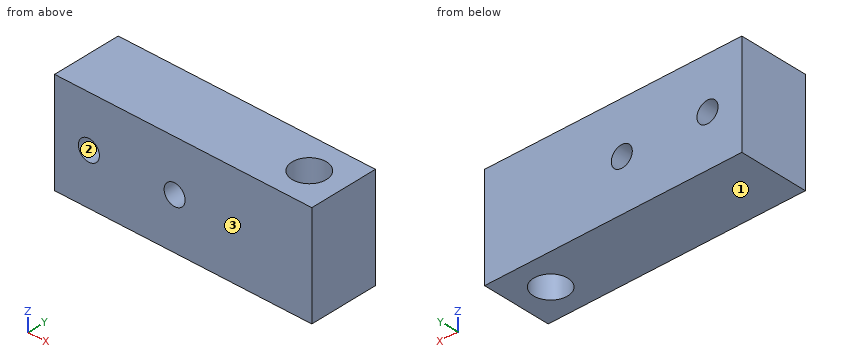
Autodesk Inventor part; units mm, degrees
ref_plane "YZ Plane" through (0, 0, 0) normal (1, 0, 0) x (0, 1, 0)
ref_plane "XZ Plane" through (0, 0, 0) normal (0, 1, 0) x (-1, 0, 0)
ref_plane "XY Plane" through (0, 0, 0) normal (0, 0, 1) x (1, 0, 0)
sketch "Sketch1" plane through (0, 0, 0) normal (0, 0, 1) x (1, 0, 0)
  line L0 (0, 0) -> (95.25, 0)
  line L1 (95.25, 0) -> (95.25, 25.4)
  line L2 (95.25, 25.4) -> (0, 25.4)
  line L3 (0, 25.4) -> (0, 0)
  circle A0 centre (82.55, 12.7) radius 6.35
  dimension "d0" = 25.4
  dimension "d1" = 95.25
  dimension "d2" = 12.7
  dimension "d3" = 12.7
  dimension "d4" = 12.7
extrude "Extrusion1" add sketch "Sketch1" along normal blind 38.1
hole "Hole1" at (12.7, 25.4, 19.05) direction (0, -1, 0) diameter 7.7978 end through all
pattern_linear "Rectangular Pattern1" count 2 spacing 31.75 along (1, 0, 0) of "Hole1"
equation "\"d3\" = 0.5 * d0"
equation "\"d4\" = d3"
properties part number "GE-12023"
Work out the finished part from the listing and answer in its coordinate system (mm). Face numbers are marked on the shaded views. Give positions to 0.01 mm unless a question says otherwise; leave off trailing zeros. Order: outer loops, then holes, each group sorted by start corner. A loop starts at its lowest first (then second) coordinate and runs counter-clockwise, first axis right, second up. Notation, with made-up numbers: (36.25, 89) - (49.25, 89) arc R29 cw to (49.25, 127) - close; hole circle Ø6 at (69.25, 38). An arc over 180 degrees is marked (long way). One line per item, written item: value. Start each with the question number.
1. Section A-A, the plane y = 12.7 is taken. Write down the section's boundary in (x, z), then the cut area to 3 significant figures.
2. Section D-D, the plane y = 3.5 is taken. Write down the section's boundary in (x, z).
3. For a pull along Z with two mould halves and no side action, classify the marked faces 1, 2 and 3 as released by +Z, released by -Z, zero draft, split by the parting line, or undercut.
4. Section C-C, the plane z = 19.05 is taken. Write down the section's boundary in (x, y).
5. Consider line 1 (Z direction, x = 12.7, y = 9); line 2 (X direction, y = 10.75, z = 19.05); line 3 (Y direction, x = 83, z = 13.5). Determine where each line is inside the solid, lowest interval first.
6. Section B-B, the plane x = 44.45 is taken. Write down the section's boundary in (y, z).
Filled sheet:
1. outline: (0, 0) - (76.2, 0) - (76.2, 38.1) - (0, 38.1) - close; (88.9, 0) - (95.25, 0) - (95.25, 38.1) - (88.9, 38.1) - close; hole circle Ø7.8 at (12.7, 19.05); hole circle Ø7.8 at (44.45, 19.05)
1. area: 3,050 mm²
2. outline: (0, 0) - (95.25, 0) - (95.25, 38.1) - (0, 38.1) - close; hole circle Ø7.8 at (12.7, 19.05); hole circle Ø7.8 at (44.45, 19.05)
3. face 1: released by -Z
3. face 2: undercut
3. face 3: zero draft
4. outline: (0, 0) - (8.8, 0) - (8.8, 25.4) - (0, 25.4) - close; (16.6, 0) - (40.55, 0) - (40.55, 25.4) - (16.6, 25.4) - close; (48.35, 0) - (95.25, 0) - (95.25, 25.4) - (48.35, 25.4) - close; hole circle Ø12.7 at (82.55, 12.7)
5. line 1: 0 to 15.15, 22.95 to 38.1
5. line 2: 0 to 8.8, 16.6 to 40.55, 48.35 to 76.51, 88.59 to 95.25
5. line 3: 0 to 6.37, 19.03 to 25.4
6. outline: (0, 0) - (25.4, 0) - (25.4, 15.15) - (0, 15.15) - close; (0, 22.95) - (25.4, 22.95) - (25.4, 38.1) - (0, 38.1) - close
